from build123d import *

# Parameters (mm, degrees)
CYLINDER2163_R               = 1.5
CYLINDER2163_DEPTH           = 100
CYLINDER2164_R               = 1.5
CYLINDER2164_DEPTH           = 100
CYLINDER2164_PLACEMENT_ANGLE = 145
CYLINDER2165_R               = 1.5
CYLINDER2165_DEPTH           = 100
CYLINDER2166_R               = 1.5
CYLINDER2166_DEPTH           = 100
CYLINDER2166_PLACEMENT_ANGLE = 225
CYLINDER2167_R               = 1.5
CYLINDER2167_DEPTH           = 100
CYLINDER2168_R               = 1.5
CYLINDER2168_DEPTH           = 100
CYLINDER2168_PLACEMENT_ANGLE = 45
CYLINDER2162_R               = 1.5
CYLINDER2162_DEPTH           = 100
CYLINDER2161_R               = 1.5
CYLINDER2161_DEPTH           = 100
CYLINDER2161_PLACEMENT_ANGLE = 45
TUBE089_R                    = 58
TUBE089_R_2                  = 32
TUBE089_DEPTH                = 1


with BuildPart() as obj1:
    # Cylinder2163 → Cylinder2163 (new body)
    with BuildSketch(Plane(origin=(38, 0, 0), x_dir=(0, 1, 0), z_dir=(0, 0, 1))):
        Circle(CYLINDER2163_R)
    extrude(amount=CYLINDER2163_DEPTH)


with BuildPart() as obj2:
    # Cylinder2164 → Cylinder2164 (new body)
    with BuildSketch(Plane.XY):
        Circle(CYLINDER2164_R)
    extrude(amount=CYLINDER2164_DEPTH)


with BuildPart() as obj2_1:
    # Cylinder2164 placement: moved
    add(obj2.part.moved(Location((21.795905, 31.127778, 0))).rotate(Axis((21.795905, 31.127778, 0), (0, 0, 1)), CYLINDER2164_PLACEMENT_ANGLE))


with BuildPart() as obj3:
    # Cylinder2165 → Cylinder2165 (new body)
    with BuildSketch(Plane(origin=(0, 38, 0), x_dir=(-1, 0, 0), z_dir=(0, 0, 1))):
        Circle(CYLINDER2165_R)
    extrude(amount=CYLINDER2165_DEPTH)


with BuildPart() as obj4:
    # Cylinder2166 → Cylinder2166 (new body)
    with BuildSketch(Plane.XY):
        Circle(CYLINDER2166_R)
    extrude(amount=CYLINDER2166_DEPTH)


with BuildPart() as obj4_1:
    # Cylinder2166 placement: moved
    add(obj4.part.moved(Location((-26.870058, 26.870058, 0))).rotate(Axis((-26.870058, 26.870058, 0), (0, 0, 1)), CYLINDER2166_PLACEMENT_ANGLE))


with BuildPart() as obj5:
    # Cylinder2167 → Cylinder2167 (new body)
    with BuildSketch(Plane(origin=(-38, 0, 0), x_dir=(0, -1, 0), z_dir=(0, 0, 1))):
        Circle(CYLINDER2167_R)
    extrude(amount=CYLINDER2167_DEPTH)


with BuildPart() as obj6:
    # Cylinder2168 → Cylinder2168 (new body)
    with BuildSketch(Plane.XY):
        Circle(CYLINDER2168_R)
    extrude(amount=CYLINDER2168_DEPTH)


with BuildPart() as obj6_1:
    # Cylinder2168 placement: moved
    add(obj6.part.moved(Location((-26.870058, -26.870058, 0))).rotate(Axis((-26.870058, -26.870058, 0), (0, 0, -1)), CYLINDER2168_PLACEMENT_ANGLE))


with BuildPart() as obj7:
    # Cylinder2162 → Cylinder2162 (new body)
    with BuildSketch(Plane(origin=(0, -38, 0), x_dir=(1, 0, 0), z_dir=(0, 0, 1))):
        Circle(CYLINDER2162_R)
    extrude(amount=CYLINDER2162_DEPTH)


with BuildPart() as compound1127:
    # Cylinder2161 → Cylinder2161 (new body)
    with BuildSketch(Plane.XY):
        Circle(CYLINDER2161_R)
    extrude(amount=CYLINDER2161_DEPTH)


with BuildPart() as compound1127_1:
    # Cylinder2161 placement: moved
    add(compound1127.part.moved(Location((26.870058, -26.870058, 0))).rotate(Axis((26.870058, -26.870058, 0), (0, 0, 1)), CYLINDER2161_PLACEMENT_ANGLE))

    # Compound1127: union obj1, obj2, obj3, obj4, obj5, obj6, obj7
    add(obj1.part)
    add(obj2_1.part)
    add(obj3.part)
    add(obj4_1.part)
    add(obj5.part)
    add(obj6_1.part)
    add(obj7.part)


with BuildPart() as cut715:
    # Tube089 → Tube089 (new body)
    with BuildSketch(Plane.XY.offset(42)):
        Circle(TUBE089_R)
        Circle(TUBE089_R_2, mode=Mode.SUBTRACT)
    extrude(amount=TUBE089_DEPTH)

    # Cut715: cut Compound1127
    add(compound1127_1.part, mode=Mode.SUBTRACT)


solid = cut715.part
For this review, take the finished solid that the model builds, in its own axes (mm). Coordinates: 2 decimals unless noted, no trailing zeros. Write each loop counter-clockwise with the first axis right and the second up, starting at its lowest first coordinate (ties: lowest second). Pieces come first, ordered by that corner, then holes. Notation, with made-up numbers: (18, -15.75) -> (31, -15.75) arc R8 ccw to (31, -8.75) -> close; hole circle Ø10 at (72.25, -30). An arc over 180 degrees is marked (long way). Write each question's results on one line, items separated by ' | '. Start each with the question number.
1) Wall thickness on L1, parallel to Y at x = 1, z = 42.3; L2, parallel to Y at x = -28, z = 42.5; L3, parallel to X at y = 14.5, z = 42.95: over which ranges is each line inside the solid? List them lowest first. Write a range as [from, to].
2) Insertion check: pin 1 (2.5 mm diameter, centred on x = 26.87, y = -26.87, fed in from +Z). The pin has a flat end and moves straight along its axis. Give the tip position at first contact, or say it passes through.
3) The part is to be moulded in two halves that separate along X. For faces 1 (the face through (25, -25, 42)), 2 (the face through (26.76, -51.46, 42.49)), 3 (the face through (39.464, -0.325, 42.493)), say which applies: +X half, -X half, draft (parallel to the pull), parting line (faces both ways), or undercut.
4) Consider section B-B (x = -38). Write out the cut boundary in (y, z), plus the area to 3 significant figures.
5) Consider section A-A (y = 0). Write out the cut boundary in (x, z), plus the area to 3 significant figures.
Geometry says:
1) L1: [-57.99, -39.12], [-36.88, -31.98], [31.98, 36.88], [39.12, 57.99] | L2: [-50.79, -27.86], [-25.88, -15.49], [15.49, 25.88], [27.86, 50.79] | L3: [-56.16, -28.53], [28.53, 56.16]
2) pin 1: through
3) face 1: draft | face 2: parting line | face 3: undercut
4) outline: (-43.82, 42) -> (-1.5, 42) -> (-1.5, 43) -> (-43.82, 43) -> close; (1.5, 42) -> (43.82, 42) -> (43.82, 43) -> (1.5, 43) -> close | area: 84.6 mm^2
5) outline: (-58, 42) -> (-39.5, 42) -> (-39.5, 43) -> (-58, 43) -> close; (-36.5, 42) -> (-32, 42) -> (-32, 43) -> (-36.5, 43) -> close; (32, 42) -> (36.5, 42) -> (36.5, 43) -> (32, 43) -> close; (39.5, 42) -> (58, 42) -> (58, 43) -> (39.5, 43) -> close | area: 46.0 mm^2
